Source: three-view drawing plus pictorial views. Frame: mm from the lowest corner of the part. Coordinates: 2 decimals unless noted, no trailing zeros. Order: outer loops, then holes, each group sorted by start corner. A loop starts at its lowest first (then second) coordinate and runs counter-clockwise, first axis right, second up. Notation, with made-up numbers: M -21.75,8 L 9.25,8 A12 ccw 9.25,30 Z; hole C 57,29 d3. An arc over 180 degrees is marked long. Write item = value, one per line. Start each with the question number.
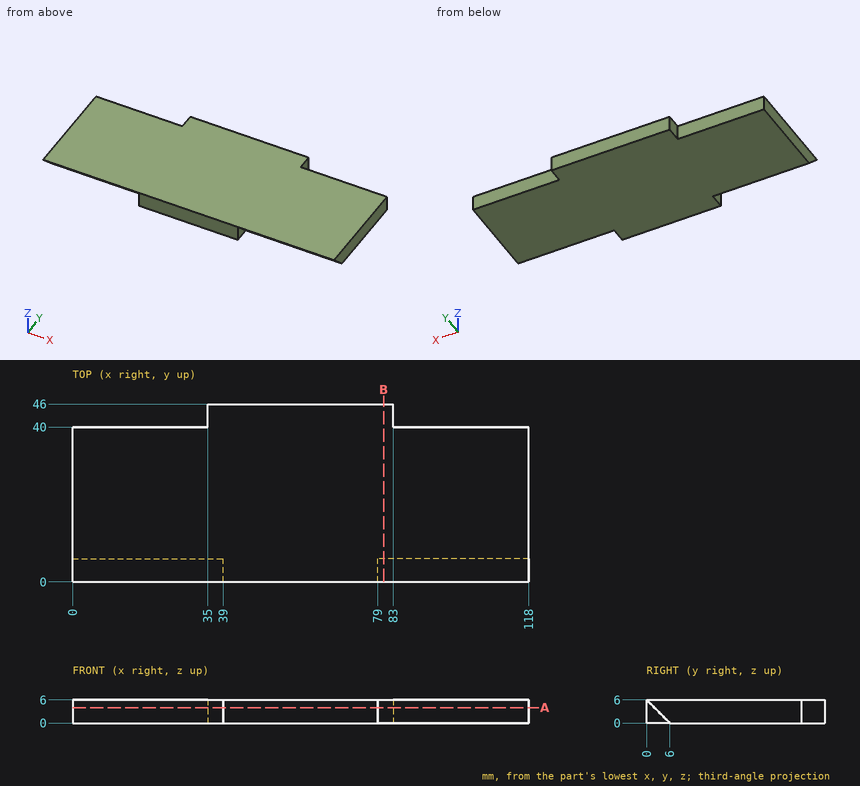
Item 1: Section query A-A on z = 4. Output: boundary loops of the cut face in (x, y), and give its area (3 significant figures).
Item 2: Section query B-B on x = 80.5. Output: boundary loops of the cut face in (y, z).
Item 3: First-contact query: pin 1 (1.8 mm diameter, centred on y = 44.5, z = 2, fed in from +X); pin 2 (3 mm diameter, centred on x = 21.5, z = 2.5, fed in from +Y). Flat tips, straight axial feed; report the tip coordinate or a pass-through.
Item 4: Material intervals for probe 1 along X at (y, z) = (41, 5.5); probe 2 along Y at (x, z) = (103.5, 4.75); probe 3 along X at (y, z) = (4.5, 1), sorted ascending. Write a range as [from, to].
Ans:
q1.outline = M 0,2 L 39,2 L 39,0 L 79,0 L 79,2 L 118,2 L 118,40 L 83,40 L 83,46 L 35,46 L 35,40 L 0,40 Z
q1.area = 4,850 mm^2
q2.outline = M 0,6 L 6,0 L 46,0 L 46,6 Z
q3.pin_1 = 83
q3.pin_2 = 40
q4.probe_1 = [35, 83]
q4.probe_2 = [1.25, 40]
q4.probe_3 = [39, 79]
